Input: dimensioned drawing with shaded views. Units: mm. Origin: part minimum x, y, z. Round coordinates to 2 decimals unless told otherwise and drop trailing zeros. Order: outer loops, then holes, each group sorted by start corner. A loop starts at its lowest first (then second) coordinate and runs counter-clockwise, first axis right, second up. Notation, with made-up numbers: (56, 80) - (99, 80) arc R22 cw to (99, 109) - close; hole circle Ø11 at (28, 39.25). An arc over 180 degrees is marked (long way). Return JSON: item names as keys, results as strings. Group by question number.
1) Ray query, line 1 (Z direction, x = 2, y = 2.15); line 2 (X direction, y = 1.95, z = 11.75) (1 decimal); line 3 (X direction, y = 1.55, z = 3.5). Return the intervals inside material, ascending. Write a range as from..to.
2) Section A-A, the plane z = 11.25. Return loops of the section in (x, y), plus the area to 3 significant figures.
3) Contact query for flat-ended pins moving along their axis: P1, Ø6, axis at x = 14, z = 6, coming from the -Y side; P2, Ø1.8, axis at x = 2.54, z = 12.24, coming from the +Y side. Output: stop coordinate, or through.
4) Section C-C, the plane x = 2.54. Return loops of the section in (y, z), plus the area to 3 significant figures.
5) Section B-B, the plane y = 0.4. Return loops of the section in (x, z), plus the area to 3 significant figures.
6) Mould query, pull axis X, two halves, no side actions, for the marked faces 1, 2 and 3. Classes: pulls with the +X half, pulls with the -X half, needs draft (parallel to the pull), parting line crosses it, or undercut.
7) Section D-D, the plane z = 2.75. Return loops of the section in (x, y).
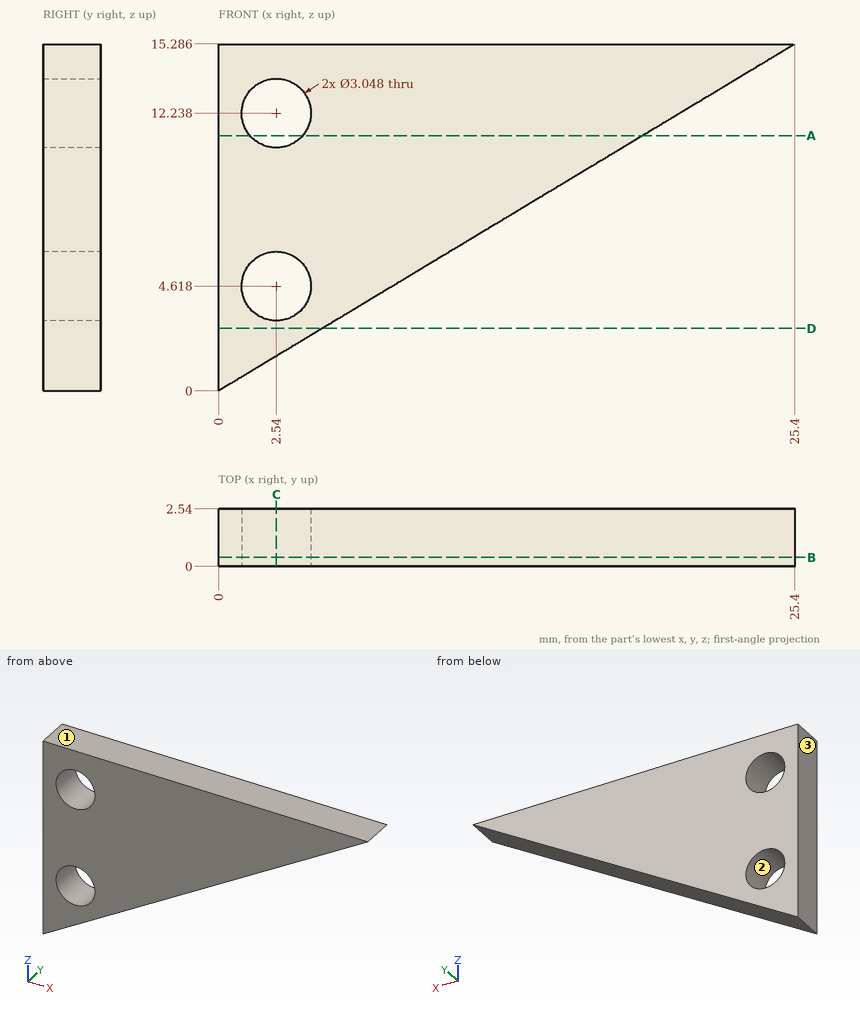
Geometry check:
{
 "1": {"line 1": "1.2..3.19, 6.04..10.81, 13.66..15.29", "line 2": "0..1.1, 4..19.5", "line 3": "0..1.5, 3.58..5.82"},
 "2": {"outline": "(0, 0) - (1.38, 0) - (1.38, 2.54) - (0, 2.54) - close; (3.7, 0) - (18.69, 0) - (18.69, 2.54) - (3.7, 2.54) - close", "area": "41.6 mm2"},
 "3": {"P1": "y = 0", "P2": "through"},
 "4": {"outline": "(0, 1.53) - (2.54, 1.53) - (2.54, 3.09) - (0, 3.09) - close; (0, 6.14) - (2.54, 6.14) - (2.54, 10.71) - (0, 10.71) - close; (0, 13.76) - (2.54, 13.76) - (2.54, 15.29) - (0, 15.29) - close", "area": "19.5 mm2"},
 "5": {"outline": "(0, 0) - (25.4, 15.29) - (0, 15.29) - close; hole circle Ø3.05 at (2.54, 4.62); hole circle Ø3.05 at (2.54, 12.24)", "area": "180 mm2"},
 "6": {"face 1": "needs draft", "face 2": "undercut", "face 3": "pulls with the -X half"},
 "7": {"outline": "(0, 0) - (4.57, 0) - (4.57, 2.54) - (0, 2.54) - close"}
}
